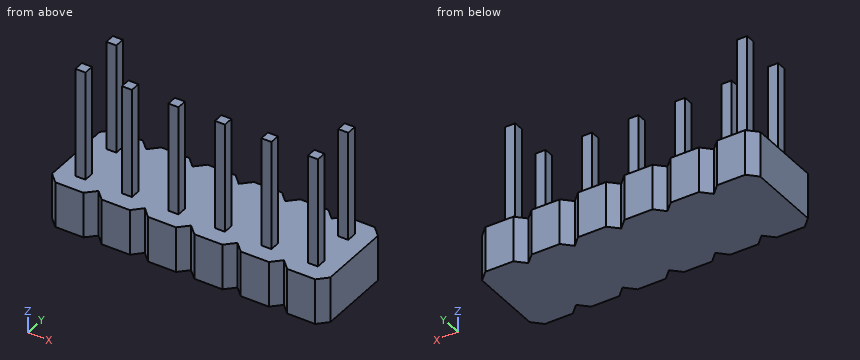
from build123d import *

# Parameters (mm, degrees)
BOSS_EXTRUDE1_DEPTH = 2.5
SKETCH2_W           = 0.55
SKETCH2_H           = 0.55
BOSS_EXTRUDE2_DEPTH = 6


with BuildPart() as part:
    # Sketch1 → Boss-Extrude1 (new body)
    with BuildSketch(Plane.XY):
        Polygon((0, 0), (0, 4), (0.502045815, 4.502045815), (2.042045815, 4.502045815), (2.546129141, 4.002045815), (3.046129141, 4.502045815), (4.586129141, 4.502045815), (5.086129141, 4.002045815), (5.586129141, 4.502045815), (7.126129141, 4.502045815), (7.626129141, 4.002045815), (8.130212468, 4.502045815), (9.670212468, 4.502045815), (10.172258282, 4), (10.674304097, 4.502045815), (12.214304097, 4.502045815), (12.718387423, 4.002045815), (13.218387423, 4.502045815), (14.758387423, 4.502045815), (15.258387423, 4.002045815), (15.258387423, 0.006055212), (14.76247075, -0.502045815), (13.22247075, -0.502045815), (12.718387423, -0.002045815), (12.214304097, -0.502045815), (10.674304097, -0.502045815), (10.172258282, 0), (9.670212468, -0.502045815), (8.130212468, -0.502045815), (7.626129141, -0.002045815), (7.122045815, -0.502045815), (5.582045815, -0.502045815), (5.086129141, 0.006055212), (4.590212468, -0.502045815), (3.050212468, -0.502045815), (2.546129141, -0.002045815), (2.042045815, -0.502045815), (0.502045815, -0.502045815), align=None)
    extrude(amount=BOSS_EXTRUDE1_DEPTH)

    # Sketch2 → Boss-Extrude2 (add)
    with BuildSketch(Plane.XY.offset(2.5)):
        with Locations((1.275, 0.702954185)):
            Rectangle(SKETCH2_W, SKETCH2_H)
        with Locations((1.275, 3.297045815)):
            Rectangle(SKETCH2_W, SKETCH2_H)
        with Locations((3.825, 0.702954185)):
            Rectangle(SKETCH2_W, SKETCH2_H)
        with Locations((6.375, 0.702954185)):
            Rectangle(SKETCH2_W, SKETCH2_H)
        with Locations((8.925, 0.702954185)):
            Rectangle(SKETCH2_W, SKETCH2_H)
        with Locations((11.475, 0.702954185)):
            Rectangle(SKETCH2_W, SKETCH2_H)
        with Locations((14.025, 0.702954185)):
            Rectangle(SKETCH2_W, SKETCH2_H)
        with Locations((14.025, 3.252954185)):
            Rectangle(SKETCH2_W, SKETCH2_H)
    extrude(amount=BOSS_EXTRUDE2_DEPTH)


solid = part.part
Part model, mm, in its own coordinate system. Give positions to 0.01 mm unless a question says otherwise; leave off trailing zeros. Loops run counter-clockwise (first coordinate to the right, second up) from the corner with the lowest first, then second, coordinate; pieces in that order, holes last.
(1) Drill centre lines: line 1 along X through (y, z) = (3.1, 5.25); line 2 along X through (y, z) = (0.5, 3.5); line 3 along Y through (x, z) = (1.5, 5.5). Where is each one in solid material? Low to high.
Return value:
line 1: x = 1 to 1.55, 13.75 to 14.3
line 2: x = 1 to 1.55, 3.55 to 4.1, 6.1 to 6.65, 8.65 to 9.2, 11.2 to 11.75, 13.75 to 14.3
line 3: y = 0.43 to 0.98, 3.02 to 3.57
(2) Pin check, flat tips, straight feed: pin 1 (0.6 mm diameter, centred on x = 4, z = 7, fed in from -Y); pin 2 (3 mm diameter, centred on x = 6, z = 4.5, fed in from +Y); pin 3 (0.6 mm diameter, centred on y = 0.5, z = 5.5, fed in from -X). Stop position of each tip, or through.
Return value:
pin 1: stops at y = 0.43
pin 2: stops at y = 0.98
pin 3: stops at x = 1
(3) Band-saw the part on A-A (z = 6). Count the separate pieces of the cut face and the enclosed holes in it, and give its area (3 significant figures).
Return value:
separate pieces: 8
enclosed holes: 0
area: 2.42 mm2
(4) Band-saw the part on C-C (y = 4.15). Write the cut outline in (x, z).
Return value:
outline: (0.15, 0) - (2.4, 0) - (2.4, 2.5) - (0.15, 2.5) - close; (2.69, 0) - (4.94, 0) - (4.94, 2.5) - (2.69, 2.5) - close; (5.23, 0) - (7.48, 0) - (7.48, 2.5) - (5.23, 2.5) - close; (7.78, 0) - (10.02, 0) - (10.02, 2.5) - (7.78, 2.5) - close; (10.32, 0) - (12.57, 0) - (12.57, 2.5) - (10.32, 2.5) - close; (12.87, 0) - (15.11, 0) - (15.11, 2.5) - (12.87, 2.5) - close
(5) Band-saw the part on D-D (y = 2.75). Write the cut outline in (x, z), and give its area (3 significant figures).
Return value:
outline: (0, 0) - (15.26, 0) - (15.26, 2.5) - (0, 2.5) - close
area: 38.1 mm2
(6) Band-saw the part on B-B (x = 6.5). Write the cut outline in (y, z), and give its area (3 significant figures).
Return value:
outline: (-0.5, 0) - (4.5, 0) - (4.5, 2.5) - (0.98, 2.5) - (0.98, 8.5) - (0.43, 8.5) - (0.43, 2.5) - (-0.5, 2.5) - close
area: 15.8 mm2
